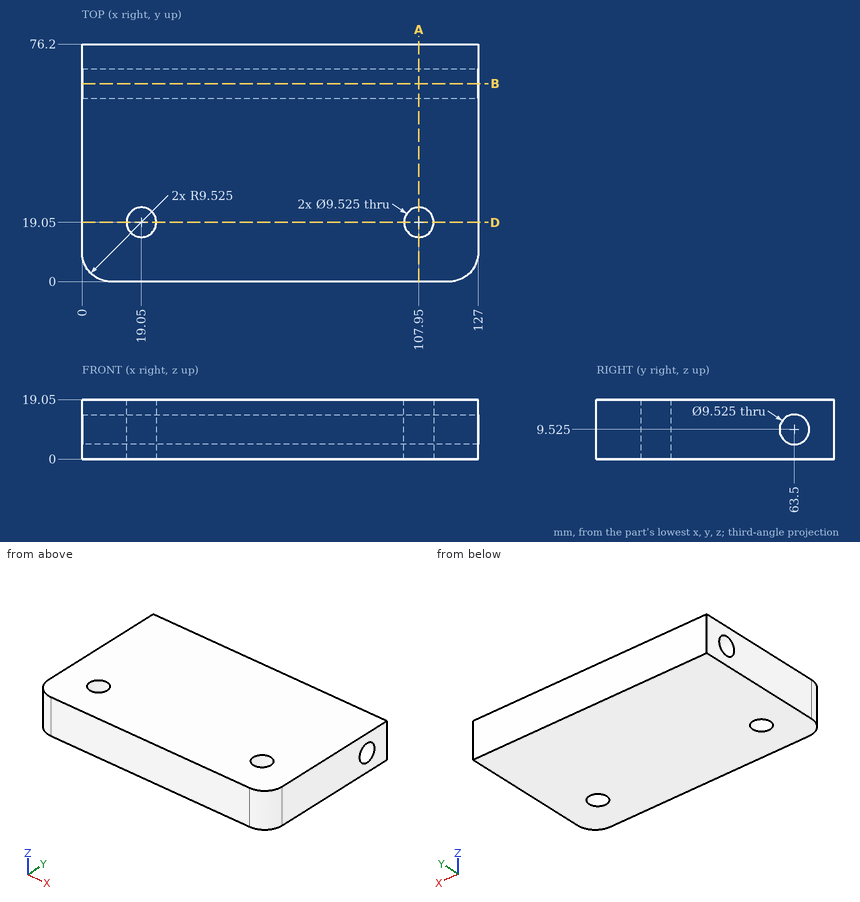
Job drawing, mm, ordinate dimensions from the low corner. One solid piece. Give positions to 0.01 mm unless a question says otherwise; leave off trailing zeros. Loops run counter-clockwise (first coordinate to the right, second up) from the corner with the lowest first, then second, coordinate; pieces in that order, holes last. Notation, with made-up numbers: (26.5, 79.5) -> (44.5, 79.5) arc R23 ccw to (44.5, 106.5) -> close; hole circle Ø4 at (68.5, 65.5). An arc over 180 degrees is marked (long way). Use a Markdown table: item, result. Add a question column.
(1) Wall check: line 1 along Z through (x, y) = (60, 63); line 2 along Y through (x, z) = (107.95, 6.75); line 3 along X through (y, z) = (17, 6.5). Give the ranges that are in metal, low to high.
(2) Slice it at D-D on y = 19.05. List the corners of the cut face in (x, z), and give its area (3 significant figures).
(3) Slice it at B-B on y = 63.5. List the corners of the cut face in (x, z), and give its area (3 significant figures).
(4) Drop a flat-ended pin along its axis: pin 1 Ø10 at (x, z) = (105.5, 4) entering from -Y. Give the stop position or say it passes through.
(5) Slice it at A-A on x = 107.95. Give the number of separate pieces and of enclosed holes in the cut face, and give its area (3 significant figures).
Filled sheet:
| question | item | result |
|---|---|---|
| 1 | line 1 | 0 to 4.79, 14.26 to 19.05 |
| 1 | line 2 | 0 to 14.29, 23.81 to 59.63, 67.37 to 76.2 |
| 1 | line 3 | 0 to 14.75, 23.35 to 103.65, 112.25 to 127 |
| 2 | outline | (0, 0) -> (14.29, 0) -> (14.29, 19.05) -> (0, 19.05) -> close; (23.81, 0) -> (103.19, 0) -> (103.19, 19.05) -> (23.81, 19.05) -> close; (112.71, 0) -> (127, 0) -> (127, 19.05) -> (112.71, 19.05) -> close |
| 2 | area | 2,060 mm2 |
| 3 | outline | (0, 0) -> (127, 0) -> (127, 4.76) -> (0, 4.76) -> close; (0, 14.29) -> (127, 14.29) -> (127, 19.05) -> (0, 19.05) -> close |
| 3 | area | 1,210 mm2 |
| 4 | pin 1 | y = 0 |
| 5 | separate pieces | 2 |
| 5 | enclosed holes | 1 |
| 5 | area | 1,200 mm2 |
